Geometry check sheet. Reference: the model listing, model coordinates, mm. A direction names the side the tool comes from. Round coordinates to 2 decimals unless told otherwise and drop trailing zeros. Loops run counter-clockwise (first coordinate to the right, second up) from the corner with the lowest first, then second, coordinate; pieces in that order, holes last. Notation, with made-up numbers: (44, 89) - (101, 89) arc R19 ccw to (101, 123) - close; hole circle Ø11 at (81.5, -9.5). An arc over 180 degrees is marked (long way). Write item = value, one per line.
```python
from build123d import *

# Parameters (mm, degrees)
F1_DEPTH = 3.175
F2_DEPTH = 3.9624
F3_R     = 2.54
F4_R     = 0.508


with BuildPart() as f1:
    # F0 (on Top) → F1 (new body)
    with BuildSketch(Plane.XY):
        Polygon((-63.5, -19.05), (63.5, -19.05), (63.5, 3.175), (-50.8, 3.175), (-50.8, 19.05), (-63.5, 19.05), align=None)
    extrude(amount=F1_DEPTH)

    # F0 (on Top) → F2 (join)
    with BuildSketch(Plane.XY):
        Polygon((63.652039, -19.05), (63.5, -19.05), (-63.5, -19.05), (-63.5, -41.275), (50.8, -41.275), (50.8, -57.15), (63.652039, -57.15), align=None)
    extrude(amount=F2_DEPTH)

    # F3
    f3_edges = [f1.edges().sort_by_distance(p)[0] for p in [
        (-63.5, -41.275, 1.9812),
        (50.8, -41.275, 1.9812),
        (50.8, -57.15, 1.9812),
        (63.652039, -57.15, 1.9812),
        (63.5, 3.175, 1.5875),
        (-50.8, 3.175, 1.5875),
        (-50.8, 19.05, 1.5875),
        (-63.5, 19.05, 1.5875),
    ]]
    fillet(f3_edges, radius=F3_R)

    # F4
    f4_edges = [f1.edges().sort_by_distance(p)[0] for p in [
        (-63.5, -28.8925, 3.9624),
        (-62.756051, -40.531051, 3.9624),
        (0.076019, -19.05, 3.9624),
        (-6.35, -41.275, 3.9624),
        (63.652039, -36.83, 3.9624),
        (50.056051, -42.018949, 3.9624),
        (62.90809, -56.406051, 3.9624),
        (50.8, -49.2125, 3.9624),
        (57.226019, -57.15, 3.9624),
        (51.543949, -56.406051, 3.9624),
        (63.5, -9.2075, 3.175),
        (63.5, -9.2075, 0),
        (62.756051, 2.431051, 0),
        (63.576019, -19.05, 0),
        (6.35, 3.175, 0),
        (63.652039, -36.83, 0),
        (-50.056051, 3.918949, 0),
        (62.90809, -56.406051, 0),
        (-50.8, 11.1125, 0),
        (57.226019, -57.15, 0),
        (-51.543949, 18.306051, 0),
        (51.543949, -56.406051, 0),
        (-57.15, 19.05, 0),
        (50.8, -49.2125, 0),
        (-62.756051, 18.306051, 0),
        (50.056051, -42.018949, 0),
        (-63.5, -11.1125, 0),
        (-6.35, -41.275, 0),
        (-62.756051, -40.531051, 0),
    ]]
    fillet(f4_edges, radius=F4_R)


solid = f1.part
```
(1) Section check B-B (x = 38). Enter the section's corners in (y, z) (3 decimals), then the cut area to 3 significant figures.
Answers follow:
outline = (-41.275, 0.508) arc R0.508 ccw to (-40.767, 0) - (2.667, 0) arc R0.508 ccw to (3.175, 0.508) - (3.175, 2.667) arc R0.508 ccw to (2.667, 3.175) - (-19.05, 3.175) - (-19.05, 3.454) arc R0.508 ccw to (-19.558, 3.962) - (-40.767, 3.962) arc R0.508 ccw to (-41.275, 3.454) - close
area = 158 mm²
(2) Section check D-D (y = -50). Enter the section's corners in (x, z), then the cut area to 3 significant figures.
Answers follow:
outline = (50.8, 0.51) arc R0.51 ccw to (51.31, 0) - (63.14, 0) arc R0.51 ccw to (63.65, 0.51) - (63.65, 3.45) arc R0.51 ccw to (63.14, 3.96) - (51.31, 3.96) arc R0.51 ccw to (50.8, 3.45) - close
area = 50.7 mm²
(3) Section check A-A (z = 2). Enter the section's corners in (x, y) (3 decimals), then the cut area to 3 significant figures.
Answers follow:
outline = (-63.5, -38.735) arc R2.54 ccw to (-60.96, -41.275) - (48.26, -41.275) arc R2.54 cw to (50.8, -43.815) - (50.8, -54.61) arc R2.54 ccw to (53.34, -57.15) - (61.112, -57.15) arc R2.54 ccw to (63.652, -54.61) - (63.652, -19.05) - (63.5, -19.05) - (63.5, 0.635) arc R2.54 ccw to (60.96, 3.175) - (-48.26, 3.175) arc R2.54 cw to (-50.8, 5.715) - (-50.8, 16.51) arc R2.54 ccw to (-53.34, 19.05) - (-60.96, 19.05) arc R2.54 ccw to (-63.5, 16.51) - close
area = 6,050 mm²
(4) Scan lines: L1, parallel to Y at x = -17.5, z = 0.6 (3 decimals); L2, parallel to X at y = -48, z = 1.3; L3, parallel to Z at x = -25, y = -17 (3 decimals). Record each from-to range of solid material in increasing order. Write a range as [from, to].
Answers follow:
L1 = [-41.275, 3.175]
L2 = [50.8, 63.65]
L3 = [0, 3.175]
(5) Set-up check for faces 1 (the cylindrical face through (-50.076, 3.939, 1.603)), 2 (the flat face through (-7, -41.275, 2)), 3 (the flat face through (-1, -8, 3.175)): record each of +Z, -Z, +X, -X, +Y, -Y from which the full face is reachable in a straight line by a thin tool's end or side.
Answers follow:
face_1 = +Z, -Z, +X, +Y
face_2 = +Z, -Z, -X, -Y
face_3 = +Z, +X, -X, +Y
(6) Gauge pin test, flat ends, axial feed: pin 1 (1.1 mm diameter, centred on x = -17, z = 1, fed in from +Y) (3 decimals); pin 2 (1 mm diameter, centred on x = 13.5, z = 2, fed in from -Y) (3 decimals); pin 3 (8 mm diameter, centred on x = 12, y = 0.5, fed in from +Z) (3 decimals). Record the tip position at first contact, or that the pin passes through.
Answers follow:
pin_1 = 3.175
pin_2 = -41.275
pin_3 = 3.175
(7) Section check C-C (y = -6). Enter the section's corners in (x, z) (3 decimals).
Answers follow:
outline = (-63.5, 0.508) arc R0.508 ccw to (-62.992, 0) - (62.992, 0) arc R0.508 ccw to (63.5, 0.508) - (63.5, 2.667) arc R0.508 ccw to (62.992, 3.175) - (-62.992, 3.175) arc R0.508 ccw to (-63.5, 2.667) - close
